Design review of the part built by this model. Coordinates are the model's own, in mm. Face numbers are marked on the shaded views. A direction names the side the tool comes from. Coordinates: 2 decimals unless noted, no trailing zeros. Write each loop counter-clockwise with the first axis right and the second up, starting at its lowest first coordinate (ties: lowest second). Pieces come first, ordered by that corner, then holes. Notation, with made-up numbers: M 35.25,51 L 46.25,51 A23 ccw 46.25,65 Z; hole C 27,65 d4. An arc over 180 degrees is marked long. Write item = value, one per line.
```python
from build123d import *

# Parameters (mm, degrees)
SKETCH1_W           = 20
SKETCH1_H           = 5.75
BOSS_EXTRUDE1_DEPTH = 17
SKETCH2_R           = 5
CUT_EXTRUDE2_DEPTH  = 7
SKETCH4_R           = 2.5
CUT_EXTRUDE3_DEPTH  = 17


with BuildPart() as part:
    # Sketch1 → Boss-Extrude1 (new body)
    with BuildSketch(Plane.XY):
        with BuildLine():
            ThreePointArc((-30.225116888, -1.226706604), (-30.119790355, -2.803699153), (-29.932240793, -4.373037976))
            Line((-29.932240793, -4.373037976), (-20.825403989, -4.226706604))
            ThreePointArc((-20.825403989, -4.226706604), (-21.073436119, -2.733640452), (-21.21456318, -1.226706604))
            Line((-21.21456318, -1.226706604), (-30.225116888, -1.226706604))
        make_face()
        with BuildLine():
            Line((-68.950810556, -1.226706604), (-68.950810556, -5))
            Line((-68.950810556, -5), (-29.932240793, -4.373037976))
            ThreePointArc((-29.932240793, -4.373037976), (-30.119790355, -2.803699153), (-30.225116888, -1.226706604))
            Line((-30.225116888, -1.226706604), (-68.950810556, -1.226706604))
        make_face()
        with BuildLine():
            Line((-68.950810556, 4.405365931), (-68.950810556, 1.405365931))
            Line((-68.950810556, 1.405365931), (-30.217336855, 1.405365931))
            ThreePointArc((-30.217336855, 1.405365931), (-30.109804839, 2.908977923), (-29.927499912, 4.405365931))
            Line((-29.927499912, 4.405365931), (-68.950810556, 4.405365931))
        make_face()
        with BuildLine():
            ThreePointArc((-29.927499912, 4.405365931), (-30.109804839, 2.908977923), (-30.217336855, 1.405365931))
            Line((-30.217336855, 1.405365931), (-21.203477229, 1.405365931))
            ThreePointArc((-21.203477229, 1.405365931), (-21.049424337, 2.91277103), (-20.788344114, 4.405365931))
            Line((-20.788344114, 4.405365931), (-29.927499912, 4.405365931))
        make_face()
        with BuildLine():
            ThreePointArc((21.25, 0), (15.0260191, -15.0260191), (0, -21.25))
            Line((0, -21.25), (10, -21.25))
            Line((10, -21.25), (14, -21.25))
            Line((14, -21.25), (14, -26.815340759))
            ThreePointArc((14, -26.815340759), (25.870470618, -15.677412095), (30.25, 0))
            ThreePointArc((30.25, 0), (2.20857733, 30.169267246), (-29.927499912, 4.405365931))
            Line((-29.927499912, 4.405365931), (-20.788344114, 4.405365931))
            ThreePointArc((-20.788344114, 4.405365931), (2.214744632, 21.134270894), (21.25, 0))
        make_face()
        with BuildLine():
            Line((-20.825403989, -4.226706604), (-29.932240793, -4.373037976))
            ThreePointArc((-29.932240793, -4.373037976), (-24.66626611, -17.511076957), (-14, -26.815340759))
            Line((-14, -26.815340759), (-14, -21.25))
            Line((-14, -21.25), (-10, -21.25))
            Line((-10, -21.25), (0, -21.25))
            ThreePointArc((0, -21.25), (-13.448884427, -16.452659592), (-20.825403989, -4.226706604))
        make_face()
        with BuildLine():
            Line((-14, -21.25), (-14, -26.815340759))
            ThreePointArc((-14, -26.815340759), (-12.03127812, -27.754474356), (-10, -28.549299466))
            Line((-10, -28.549299466), (-10, -21.25))
            Line((-10, -21.25), (-14, -21.25))
        make_face()
        with BuildLine():
            Line((10, -21.25), (0, -21.25))
            Line((0, -21.25), (-10, -21.25))
            Line((-10, -21.25), (-10, -28.549299466))
            ThreePointArc((-10, -28.549299466), (0, -30.25), (10, -28.549299466))
            Line((10, -28.549299466), (10, -21.25))
        make_face()
        with BuildLine():
            Line((14, -21.25), (10, -21.25))
            Line((10, -21.25), (10, -28.549299466))
            ThreePointArc((10, -28.549299466), (12.03127812, -27.754474356), (14, -26.815340759))
            Line((14, -26.815340759), (14, -21.25))
        make_face()
        with BuildLine():
            ThreePointArc((14, -26.815340759), (12.03127812, -27.754474356), (10, -28.549299466))
            Line((10, -28.549299466), (10, -41.310288198))
            Line((10, -41.310288198), (10, -47.060288198))
            Line((10, -47.060288198), (14, -47.060288198))
            Line((14, -47.060288198), (14, -26.815340759))
        make_face()
        with BuildLine():
            ThreePointArc((-10, -28.549299466), (-12.03127812, -27.754474356), (-14, -26.815340759))
            Line((-14, -26.815340759), (-14, -47.060288198))
            Line((-14, -47.060288198), (-10, -47.060288198))
            Line((-10, -47.060288198), (-10, -41.310288198))
            Line((-10, -41.310288198), (-10, -28.549299466))
        make_face()
        with Locations((0, -44.185288198)):
            Rectangle(SKETCH1_W, SKETCH1_H)
    extrude(amount=BOSS_EXTRUDE1_DEPTH)

    # Sketch2 → Cut-Extrude2 (cut)
    with BuildSketch(Plane.XZ.offset(47.060288198)):
        with Locations((0, 8.5)):
            Circle(SKETCH2_R)
    extrude(amount=-CUT_EXTRUDE2_DEPTH, mode=Mode.SUBTRACT)

    # Sketch4 → Cut-Extrude3 (cut)
    with BuildSketch(Plane(origin=(0.062522925, -3.89107316, 0), x_dir=(0.99987093, 0.016066225, 0), z_dir=(0.016066225, -0.99987093, 0))):
        with Locations((-49.510438917, 8.5)):
            Circle(SKETCH4_R)
        with Locations((-39.510438917, 8.5)):
            Circle(SKETCH4_R)
        with Locations((-59.510438917, 8.5)):
            Circle(SKETCH4_R)
    extrude(amount=-CUT_EXTRUDE3_DEPTH, mode=Mode.SUBTRACT)


solid = part.part
```
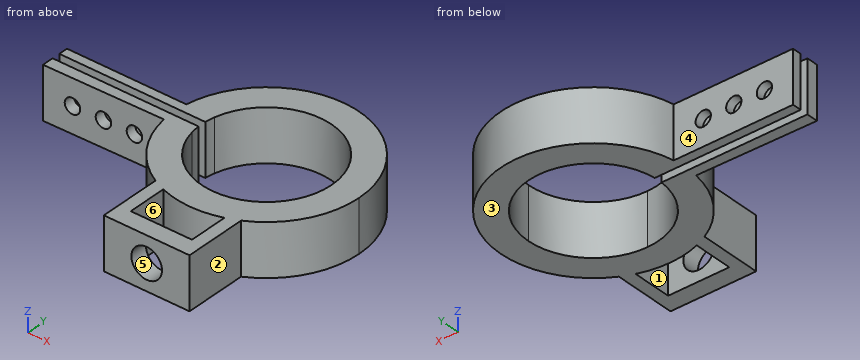
Q1. Consider section A-A, the plane y = 7. State the section outline as (x, z) points, and give its area (3 significant figures).
Check result:
outline = M -29.43,0 L -20.06,0 L -20.06,17 L -29.43,17 Z; M 20.06,0 L 29.43,0 L 29.43,17 L 20.06,17 Z
area = 318 mm²
Q2. Machinability: for the marked faces 4, 5 and 6, which of the approach directions +Z, -Z, +X, -X, +Y, -Y give a long, thin tool a straight path to every point of the face, cutting with its end or side? Answer none if there is none.
Check result:
face_4 = +Z, -Z, -X, +Y
face_5 = -Y
face_6 = +Z, -Z
Q3. Wall thickness on line 1 (Z direction, x = 0, y = -44); line 2 (Y direction, x = 7, z = 1.75); line 3 (Y direction, x = -3, z = 2): over which ranges is each line inside the solid? List them lowest first.
Check result:
line_1 = 0 to 3.5, 13.5 to 17
line_2 = -47.06 to -41.31, -29.43 to -20.06, 20.06 to 29.43
line_3 = -47.06 to -41.31, -30.1 to -21.04, 21.04 to 30.1
Q4. Consider section B-B, the plane z = 8.5. State how many separate pieces and enclosed holes the cut face has, and give its area (3 significant figures).
Check result:
separate_pieces = 7
enclosed_holes = 0
area = 1,800 mm²
Q5. The part is to be moulded in two halves that separate along X. For the marked faces 1, 2 and 3, say which applies: +X half, -X half, draft (parallel to the pull), parting line (faces both ways), or undercut.
Check result:
face_1 = undercut
face_2 = +X half
face_3 = draft
Q6. For P1, Ø4, axis at y = -35.5, z = 5, coming from the +X side; P2, Ø8.5, axis at x = -53, z = 10.5, coming from the +Y side; P3, Ø8.5, axis at y = -35.5, z = 12, coming from the -X side, all flat-tipped, find the tip position at first contact; note any pin that passes through.
Check result:
P1 = 14
P2 = 4.41
P3 = -14
